from build123d import *

# Parameters (mm, degrees)
RESSALTO_EXTRUS_O1_DEPTH = 400
ESBO_O2_R                = 5
CORTE_EXTRUS_O1_DEPTH    = 7.35


with BuildPart() as part:
    # Esboço1 → Ressalto-extrusão1 (new body)
    with BuildSketch(Plane.XY):
        with BuildLine():
            Line((-69.85, 0), (69.85, 0))
            Line((69.85, 0), (69.85, 6.35))
            Line((69.85, 6.35), (9.525, 6.35))
            ThreePointArc((9.525, 6.35), (5.034871939, 8.209871939), (3.175, 12.7))
            Line((3.175, 12.7), (3.175, 89.3))
            Line((3.175, 89.3), (-3.175, 89.3))
            Line((-3.175, 89.3), (-3.175, 12.7))
            ThreePointArc((-3.175, 12.7), (-5.034871939, 8.209871939), (-9.525, 6.35))
            Line((-9.525, 6.35), (-69.85, 6.35))
            Line((-69.85, 6.35), (-69.85, 0))
        make_face()
    extrude(amount=RESSALTO_EXTRUS_O1_DEPTH)

    # Esboço2 → Corte-extrusão1 (cut, through all)
    with BuildSketch(Plane(origin=(0, 6.35, 0), x_dir=(1, 0, 0), z_dir=(0, 1, 0))):
        with Locations((50, -75)):
            Circle(ESBO_O2_R)
        with Locations((-50, -75)):
            Circle(ESBO_O2_R)
        with Locations((50, -325)):
            Circle(ESBO_O2_R)
        with Locations((-50, -325)):
            Circle(ESBO_O2_R)
    extrude(amount=-CORTE_EXTRUS_O1_DEPTH, mode=Mode.SUBTRACT)


solid = part.part
Input: part model. Units: mm. Frame: model coordinates. A direction names the side the tool comes from. Give positions to 0.01 mm unless a question says otherwise; leave off trailing zeros. Loops run counter-clockwise (first coordinate to the right, second up) from the corner with the lowest first, then second, coordinate; pieces in that order, holes last. Notation, with made-up numbers: M -37.5,59 L -21.5,59 A20 cw -21.5,63 Z; hole C 18.5,36 d5. An arc over 180 degrees is marked long. Use CSV: the item, a comma, the result in double quotes.
(1) Section D-D, the plane y = 62. Return loops of the section in (x, z) (3 decimals), plus the area to 3 significant figures.
Outcome:
outline,"M -3.175,0 L 3.175,0 L 3.175,400 L -3.175,400 Z"
area,"2,540 mm²"
(2) Pin query (flat end, axial travel): P1, Ø6, axis at y = 79.5, z = 228.5, coming from the +X side (3 decimals); P2, Ø18, axis at x = -38, z = 193.5, coming from the +Y side; P3, Ø1.5, axis at y = 12.5, z = 43, coming from the -X side. Return the tip coordinate at first contact, or that it passes through.
Outcome:
P1,"stops at x = 3.175"
P2,"stops at y = 6.35"
P3,"stops at x = -3.25"
(3) Section A-A, the plane x = 50. Return loops of the section in (y, z).
Outcome:
outline,"M 0,0 L 6.35,0 L 6.35,70 L 0,70 Z; M 0,80 L 6.35,80 L 6.35,320 L 0,320 Z; M 0,330 L 6.35,330 L 6.35,400 L 0,400 Z"
(4) Section B-B, the plane z = 325. Return loops of the section in (x, y) (3 decimals).
Outcome:
outline,"M -69.85,0 L -55,0 L -55,6.35 L -69.85,6.35 Z; M -45,0 L 45,0 L 45,6.35 L 9.525,6.35 A6.35 cw 3.175,12.7 L 3.175,89.3 L -3.175,89.3 L -3.175,12.7 A6.35 cw -9.525,6.35 L -45,6.35 Z; M 55,0 L 69.85,0 L 69.85,6.35 L 55,6.35 Z"
(5) Section C-C, the plane z = 268. Return loops of the section in (x, y) (3 decimals).
Outcome:
outline,"M -69.85,0 L 69.85,0 L 69.85,6.35 L 9.525,6.35 A6.35 cw 3.175,12.7 L 3.175,89.3 L -3.175,89.3 L -3.175,12.7 A6.35 cw -9.525,6.35 L -69.85,6.35 Z"
(6) Pull-direction query (Z, two-part tool) for faces 4 (the face through (49.349, 3.219, 320.043)), 5 (the face through (-1, 0, 197)), 6 (the face through (0, 18, 400)); classes: pulls with the +Z half, pulls with the -Z half, needs draft (parallel to the pull), parting line crosses it, or undercut.
Outcome:
face 4,"undercut"
face 5,"needs draft"
face 6,"pulls with the +Z half"
(7) Material intervals for L1, parallel to X at y = 2, z = 325; L2, parallel to Z at x = -50, y = 1; L3, parallel to X at y = 49, z = 119 (3 decimals), sorted ascending. Write a range as [from, to].
Outcome:
L1,"x = [-69.85, -55], [-45, 45], [55, 69.85]"
L2,"z = [0, 70], [80, 320], [330, 400]"
L3,"x = [-3.175, 3.175]"
(8) Set-up query: faces 1 (the face through (-50.651, 3.219, 320.043)), 2 (the face through (-3.175, 52, 197)), 3 (the face through (3.175, 50, 197)). Return all of +Z, -Z, +X, -X, +Y, -Y with unobstructed straight access to the full face (end or side cutting, diameter ignored); none if empty.
Outcome:
face 1,"+Y, -Y"
face 2,"+Z, -Z, -X, +Y"
face 3,"+Z, -Z, +X, +Y"
